from build123d import *

# Parameters (mm, degrees)
F0_R     = 3.175
F1_DEPTH = 3.048


with BuildPart() as f1:
    # F0 (on Front) → F1 (new body)
    with BuildSketch(Plane.XZ):
        with BuildLine():
            ThreePointArc((3.1097588161, -12.904249902), (10.427563759, -8.2131710978), (13.2736681226, 0))
            ThreePointArc((13.2736681226, 0), (0, 13.2736681226), (-13.2736681226, 0))
            ThreePointArc((-13.2736681226, 0), (-9.3859007407, -9.3859007407), (0, -13.2736681226))
            Line((0, -13.2736681226), (3.1097588161, -12.904249902))
        make_face()
        Circle(F0_R, mode=Mode.SUBTRACT)
        with BuildLine():
            ThreePointArc((-13.2736681226, 0), (0, 13.2736681226), (13.2736681226, 0))
            ThreePointArc((13.2736681226, 0), (10.427563759, -8.2131710978), (3.1097588161, -12.904249902))
            Line((3.1097588161, -12.904249902), (45.3863375042, -7.8820795688))
            ThreePointArc((45.3863375042, -7.8820795688), (36.5129073275, -0.0804124208), (45.2264515588, 7.8994322091))
            Line((45.2264515588, 7.8994322091), (20.5507771811, 10.3248553698))
            ThreePointArc((20.5507771811, 10.3248553698), (15.2912984453, 13.0640911975), (13.39070093, 18.6813199251))
            Line((13.39070093, 18.6813199251), (15.8501799769, 62.6126332776))
            ThreePointArc((15.8501799769, 62.6126332776), (0.5628098086, 47.6349796685), (-15.7474569047, 61.4917106696))
            Line((-15.7474569047, 61.4917106696), (-15.7474569047, 60.0759088993))
            Line((-15.7474569047, 60.0759088993), (-13.2736681226, 0))
        make_face()
        with BuildLine():
            ThreePointArc((45.2264515588, 7.8994322091), (36.5129073275, -0.0804124208), (45.3863375042, -7.8820795688))
            ThreePointArc((45.3863375042, -7.8820795688), (50.3844791342, -5.2712298048), (52.3875, 0))
            ThreePointArc((52.3875, 0), (50.3307733547, 5.3310797219), (45.2264515588, 7.8994322091))
        make_face()
        with Locations((44.45, 0)):
            Circle(F0_R, mode=Mode.SUBTRACT)
        with BuildLine():
            Line((-15.7474569047, 65.5082893304), (-15.7474569047, 61.4917106696))
            ThreePointArc((-15.7474569047, 61.4917106696), (0.5628098086, 47.6349796685), (15.8501799769, 62.6126332776))
            ThreePointArc((15.8501799769, 62.6126332776), (15.8687937811, 63.0561431161), (15.875, 63.5))
            ThreePointArc((15.875, 63.5), (15.8687937811, 63.9438568839), (15.8501799769, 64.3873667224))
            Line((15.8501799769, 64.3873667224), (15.5721686032, 66.5859666221))
            ThreePointArc((15.5721686032, 66.5859666221), (-0.5459199423, 79.3656104962), (-15.7474569047, 65.5082893304))
        make_face()
        with Locations((0, 63.5)):
            Circle(F0_R, mode=Mode.SUBTRACT)
        with BuildLine():
            Line((-9.525, 114.3), (-15.7474569047, 65.5082893304))
            ThreePointArc((-15.7474569047, 65.5082893304), (-0.5459199423, 79.3656104962), (15.5721686032, 66.5859666221))
            Line((15.5721686032, 66.5859666221), (9.5243145818, 114.4142661242))
            ThreePointArc((9.5243145818, 114.4142661242), (9.5248286439, 114.3571340899), (9.525, 114.3))
            ThreePointArc((9.525, 114.3), (0, 104.775), (-9.525, 114.3))
        make_face()
        with Locations((-3.7440145388, 100.0252)):
            Circle(F0_R, mode=Mode.SUBTRACT)
        with BuildLine():
            ThreePointArc((9.5243145818, 114.4142661242), (-0.0571340899, 123.8248286439), (-9.525, 114.3))
            ThreePointArc((-9.525, 114.3), (0, 104.775), (9.525, 114.3))
            ThreePointArc((9.525, 114.3), (9.5248286439, 114.3571340899), (9.5243145818, 114.4142661242))
        make_face()
        with Locations((0, 114.3)):
            Circle(F0_R, mode=Mode.SUBTRACT)
    extrude(amount=F1_DEPTH)


solid = f1.part
Model file for the job. Use its own axes, mm. A direction names the side the tool comes from. Round coordinates to 2 decimals unless told otherwise and drop trailing zeros. Loops run counter-clockwise (first coordinate to the right, second up) from the corner with the lowest first, then second, coordinate; pieces in that order, holes last. Notation, with made-up numbers: (88, 49) - (107, 49) arc R25 ccw to (107, 72) - close; hole circle Ø10 at (18, 82.25). An arc over 180 degrees is marked (long way). Write each question's results on one line, items separated by ' | '.
(1) Wall check: L1, parallel to Z at x = 0, y = -0.65 (3 decimals); L2, parallel to Z at x = 44.45, y = -1.3 (3 decimals); L3, parallel to Z at x = -6, y = -2.05. Give the ranges that are in metal, low to high.
Answer below:
L1: z = -13.274 to -3.175, 3.175 to 60.325, 66.675 to 111.125, 117.475 to 123.825 | L2: z = -7.993 to -3.175, 3.175 to 7.976 | L3: z = -11.84 to 97.79, 102.26 to 121.7
(2) Mould opens along Z. For faces 3 (the flat face through (-12.6, -1.5, 90.2)), 4 (the cylindrical face through (15.347, -1.503, 13)), 5 (the cylindrical face through (-0.69, -1.5, -3.1)), 6 (the flat face through (3, 0, 41)) say: released by +Z, released by -Z, zero draft, split by the parting line, or undercut.
Answer below:
face 3: released by +Z | face 4: undercut | face 5: undercut | face 6: zero draft
(3) Saw through at C-C, the plane z = 34.5. List the corners of the cut face in (x, y).
Answer below:
outline: (-14.69, -3.05) - (14.28, -3.05) - (14.28, 0) - (-14.69, 0) - close
(4) Saw through at B-B, the plane x = -5. List the corners of the cut face in (y, z).
Answer below:
outline: (-3.05, -12.3) - (0, -12.3) - (0, 97.11) - (-3.05, 97.11) - close; (-3.05, 102.94) - (0, 102.94) - (0, 122.41) - (-3.05, 122.41) - close
(5) Pin check, flat tips, straight feed: pin 1 (1.5 mm diameter, centred on y = -0.5, z = 14, fed in from +X); pin 2 (1 mm diameter, centred on y = -1, z = 60, fed in from +X). Stop position of each tip, or through.
Answer below:
pin 1: stops at x = 15.14 | pin 2: stops at x = 15.73
(6) Saw through at A-A, the plane y = -0.95. Count the separate pieces of the cut face and the enclosed holes in it, then the cut area to 3 significant figures.
Answer below:
separate pieces: 1 | enclosed holes: 5 | area: 4,130 mm^2
(7) 3-axis set-ups, long thin cutter, end or side, ignore diameter. For faces 1 (the cylindrical face through (0.152, -1.503, 123.824)), 2 (the flat face through (14.6, -1.5, 40.3)): which of +Z, -Z, +X, -X, +Y, -Y reach the whole face in a straight line?
Answer below:
face 1: +Z, +Y, -Y | face 2: +X, +Y, -Y
(8) Saw through at D-D, the plane z = 50. List the corners of the cut face in (x, y), then the cut area to 3 significant figures.
Answer below:
outline: (-15.33, -3.05) - (15.14, -3.05) - (15.14, 0) - (-15.33, 0) - close | area: 92.9 mm^2
